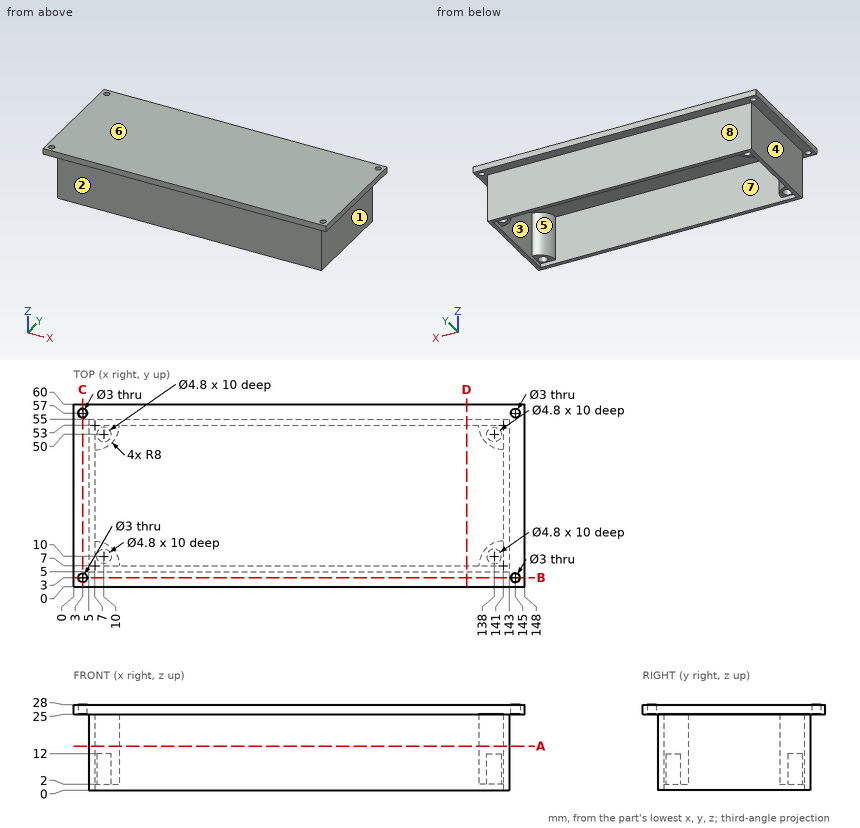
Job drawing, mm, ordinate dimensions from the low corner. One solid piece. A direction names the side the tool comes from. Round coordinates to 2 decimals unless told otherwise and drop trailing zeros. Loops run counter-clockwise (first coordinate to the right, second up) from the corner with the lowest first, then second, coordinate; pieces in that order, holes last. Notation, with made-up numbers: M 72,-23 L 127,-23 A18 ccw 127,-2 Z; hole C 55.5,34 d2. An arc over 180 degrees is marked long. One line per question, with ' | ' between items. Start each with the question number.
Item 1: Cut at B-B, the plane y = 3. Write the cut outline in (x, z).
Item 2: Pin check, flat tips, straight feed: pin 1 Ø14 at (x, y) = (90.5, 35) entering from -Z; pin 2 Ø7.5 at (x, z) = (95.5, 15) entering from -Y; pin 3 Ø1.8 at (x, y) = (145, 57) entering from -Z; pin 4 Ø1.5 at (y, z) = (52, 4) entering from +X. Stop position of each tip, or through.
Item 3: Cut at A-A, the plane z = 14.5. Write the cut outline in (x, y), plus the area to 3 significant figures.
Item 4: Cut at D-D, the plane x = 129. Write the cut outline in (y, z).
Item 5: Which spindle directions (+Z, -Z, +X, -X, +Y, -Y) get a long thin tool onto all of the face, cutting with end or side? Do the marked faces 1, 2, 3 and 4. Say none if no direction does.
Item 6: Cut at C-C, the plane x = 3. Write the cut outline in (y, z), plus the area to 3 significant figures.
Item 7: Wall check: line 1 (X direction, y = 3, z = 25.6); line 2 (Y direction, x = 145, z = 26.7); line 3 (Y direction, x = 44.5, z = 20). Give the ranges that are in metal, low to high.
Item 8: Two-plate mould, pull along Y, no slides. Class the marked faces 5, 6, 7 and 8: pulls with the +Y half, pulls with the -Y half, needs draft (parallel to the pull), parting line crosses it, or undercut.
Responses:
1) outline: M 0,25 L 1.5,25 L 1.5,28 L 0,28 Z; M 4.5,25 L 143.5,25 L 143.5,28 L 4.5,28 Z; M 146.5,25 L 148,25 L 148,28 L 146.5,28 Z
2) pin 1: stops at z = 25 | pin 2: stops at y = 5 | pin 3: passes through | pin 4: stops at x = 143
3) outline: M 5,5 L 143,5 L 143,55 L 5,55 Z; hole M 7,15 A8 cw 15,7 L 133,7 A8 cw 141,15 L 141,45 A8 cw 133,53 L 15,53 A8 cw 7,45 Z | area: 937 mm²
4) outline: M 0,25 L 5,25 L 5,0 L 7,0 L 7,25 L 53,25 L 53,0 L 55,0 L 55,25 L 60,25 L 60,28 L 0,28 Z
5) face 1: -Z, +X, +Y, -Y | face 2: -Z, +X, -X, -Y | face 3: -Z | face 4: -Z, -X, +Y, -Y
6) outline: M 0,25 L 1.5,25 L 1.5,28 L 0,28 Z; M 4.5,25 L 55.5,25 L 55.5,28 L 4.5,28 Z; M 58.5,25 L 60,25 L 60,28 L 58.5,28 Z | area: 162 mm²
7) line 1: x = 0 to 1.5, 4.5 to 143.5, 146.5 to 148 | line 2: y = 0 to 1.5, 4.5 to 55.5, 58.5 to 60 | line 3: y = 5 to 7, 53 to 55
8) face 5: undercut | face 6: needs draft | face 7: undercut | face 8: pulls with the +Y half
